```python
from build123d import *

# Parameters (mm, degrees)
SKETCH1_W           = 46
SKETCH1_H           = 31.6
BOSS_EXTRUDE1_DEPTH = 18
BOSS_EXTRUDE2_DEPTH = 3.5
SKETCH2_R           = 1.25
BOSS_EXTRUDE3_DEPTH = 5


with BuildPart() as part:
    # Sketch1 → Boss-Extrude1 (new body)
    with BuildSketch(Plane(origin=(0, 0, 0), x_dir=(1, 0, 0), z_dir=(0, 1, 0))):
        Rectangle(SKETCH1_W, SKETCH1_H)
    extrude(amount=BOSS_EXTRUDE1_DEPTH)

    # Sketch1_3 → Boss-Extrude2 (add)
    with BuildSketch(Plane(origin=(0, 0, 0), x_dir=(1, 0, 0), z_dir=(0, 1, 0))):
        with BuildLine():
            Line((-23, -6.5), (-23, 6.5))
            Line((-23, 6.5), (-30.546403177, 4.5))
            ThreePointArc((-30.546403177, 4.5), (-31.5, 3.079144467), (-30.214227812, 1.95))
            Line((-30.214227812, 1.95), (-26, 1.95))
            ThreePointArc((-26, 1.95), (-24.05, 0), (-26, -1.95))
            Line((-26, -1.95), (-30.214227812, -1.95))
            ThreePointArc((-30.214227812, -1.95), (-31.5, -3.079144467), (-30.546403177, -4.5))
            Line((-30.546403177, -4.5), (-23, -6.5))
        make_face()
        with BuildLine():
            Line((30.546403177, 4.5), (23, 6.5))
            Line((23, 6.5), (23, -6.5))
            Line((23, -6.5), (30.546403177, -4.5))
            ThreePointArc((30.546403177, -4.5), (31.5, -3.079144467), (30.214227812, -1.95))
            Line((30.214227812, -1.95), (26, -1.95))
            ThreePointArc((26, -1.95), (24.05, 0), (26, 1.95))
            Line((26, 1.95), (30.214227812, 1.95))
            ThreePointArc((30.214227812, 1.95), (31.5, 3.079144467), (30.546403177, 4.5))
        make_face()
    extrude(amount=BOSS_EXTRUDE2_DEPTH)

    # Sketch2 → Boss-Extrude3 (add)
    with BuildSketch(Plane.XY.offset(15.8)):
        with Locations((19, 13)):
            Circle(SKETCH2_R)
        with Locations((13, 13)):
            Circle(SKETCH2_R)
        with Locations((-19, 13)):
            Circle(SKETCH2_R)
        with Locations((-13, 13)):
            Circle(SKETCH2_R)
    extrude(amount=BOSS_EXTRUDE3_DEPTH)


solid = part.part
```
The model under review builds one solid part; all positions refer to its coordinate system, in mm. A direction names the side the tool comes from. Give positions to 0.01 mm unless a question says otherwise; leave off trailing zeros. Write each loop counter-clockwise with the first axis right and the second up, starting at its lowest first coordinate (ties: lowest second). Pieces come first, ordered by that corner, then holes. Notation, with made-up numbers: (-0.5, 78.5) -> (14.5, 78.5) arc R12 ccw to (14.5, 85.5) -> close; hole circle Ø3 at (67.25, -29.5). An arc over 180 degrees is marked (long way). Answer in a Markdown table with one row per item.
1) Mouldability with a two-part tool opening along Z and no side actions: class faces 6 (the cylindrical face through (24.05, 1.73, 0.04)), 7 (the flat face through (-19, 13, 20.8)), 8 (the cylindrical face through (-31.496, 1.726, 3.053)), 9 (the flat face through (24, 3.5, 1)) as +Z half, -Z half, draft (parallel to the pull), parting line (faces both ways), or undercut.
Worked answers:
| item | result |
|---|---|
| face 6 | undercut |
| face 7 | +Z half |
| face 8 | undercut |
| face 9 | draft |
2) Add section D-D on z = 13.5. State the section outline as (x, y) points.
Worked answers:
| item | result |
|---|---|
| outline | (-23, 0) -> (23, 0) -> (23, 18) -> (-23, 18) -> close |
3) Tool access review of faces 1 (the cylindrical face through (-13.16, 14.24, 18.26)), 2 (the flat face through (28, 2, -1.95)), 3 (the flat face through (-24, 3.5, 1)), 4 (the flat face through (-28, 2, 1.95)), 5 (the flat face through (-26.826, 1.726, 5.486)): name each direction out of +Z, -Z, +X, -X, +Y, -Y from which nothing blocks a thin tool from reaching the whole face with its end or side.
Worked answers:
| item | result |
|---|---|
| face 1 | +Z |
| face 2 | +X, +Y, -Y |
| face 3 | +Z, -Z, -X, +Y |
| face 4 | -X, +Y, -Y |
| face 5 | +Z, -X, +Y, -Y |
4) Add section B-B on z = 18. State the section outline as (x, y) points, plus the area to 3 significant figures.
Worked answers:
| item | result |
|---|---|
| outline | circle Ø2.5 at (-19, 13); circle Ø2.5 at (-13, 13); circle Ø2.5 at (13, 13); circle Ø2.5 at (19, 13) |
| area | 19.6 mm² |
5) Add section C-C on y = 13. State the section outline as (x, z) points.
Worked answers:
| item | result |
|---|---|
| outline | (-23, -15.8) -> (23, -15.8) -> (23, 15.8) -> (20.25, 15.8) -> (20.25, 20.8) -> (17.75, 20.8) -> (17.75, 15.8) -> (14.25, 15.8) -> (14.25, 20.8) -> (11.75, 20.8) -> (11.75, 15.8) -> (-11.75, 15.8) -> (-11.75, 20.8) -> (-14.25, 20.8) -> (-14.25, 15.8) -> (-17.75, 15.8) -> (-17.75, 20.8) -> (-20.25, 20.8) -> (-20.25, 15.8) -> (-23, 15.8) -> close |
6) Add section A-A on x = 13. State the section outline as (y, z) points.
Worked answers:
| item | result |
|---|---|
| outline | (0, -15.8) -> (18, -15.8) -> (18, 15.8) -> (14.25, 15.8) -> (14.25, 20.8) -> (11.75, 20.8) -> (11.75, 15.8) -> (0, 15.8) -> close |
7) Clearance check with flat-ended pins moving along their axes: P1, Ø1, axis at x = -28, y = 2, coming from the +Z side; P2, Ø7, axis at x = 29, z = 1.5, coming from the +Y side; P3, Ø2, axis at x = -23, z = 15.5, coming from the -Y side; P4, Ø9, axis at y = 10.5, z = -3.5, coming from the +X side. State where each tip first meets the part, or that it passes through.
Worked answers:
| item | result |
|---|---|
| P1 | z = 5.31 |
| P2 | y = 3.5 |
| P3 | y = 0 |
| P4 | x = 23 |
8) For L1, parallel to Z at x = 19, y = 1; L2, parallel to X at y = 8.75, z = -5; L3, parallel to Y at x = 18, z = 17.5, list the stretches that pass through material, from the lowest coordinate up. Write a range as [from, to].
Worked answers:
| item | result |
|---|---|
| L1 | [-15.8, 15.8] |
| L2 | [-23, 23] |
| L3 | [12.25, 13.75] |
